For this review, take the finished solid that the model builds, in its own axes (mm). A direction names the side the tool comes from. Give positions to 0.01 mm unless a question says otherwise; leave off trailing zeros. Write each loop counter-clockwise with the first axis right and the second up, starting at its lowest first coordinate (ties: lowest second). Pieces come first, ordered by that corner, then holes. Notation, with made-up numbers: M -25,10.25 L -12,10.25 A23 ccw -12,45.25 Z; hole C 87,-39.5 d10. An arc over 180 degrees is marked long. One line per item, written item: value. Start each with the question number.
Item 1: To check wall thickness, follow probe 1 along X at (y, z) = (95.5, -1); probe 2 along X at (y, z) = (13, -12.5); probe 3 along Y at (x, z) = (33.5, 21.5). State the ranges of each line that lie inside material, in increasing order.
Item 2: Tool access review of faces 3 (the face through (0, 150, 0)), 4 (the face through (6, 0, 30)): name each direction out of +Z, -Z, +X, -X, +Y, -Y from which nothing blocks a thin tool from reaching the whole face with its end or side.
Item 3: Consider section C-C, the plane y = 2. Write out the cut boundary in (x, z).
Item 4: Mouldability with a two-part tool opening along Z and no side actions: class faces 1 (the face through (0, -10, 0)), 2 (the face through (4.336, 65.216, -19.524)) as released by +Z, released by -Z, zero draft, split by the parting line, or undercut.
Item 5: Clearance check with flat-ended pins moving along their axes: pin 1 Ø1 at (y, z) = (36.5, 10.5) entering from -X; pin 2 Ø6 at (y, z) = (40, 7) entering from -X; pin 3 Ø6 at (x, y) = (-21.5, 85.5) entering from +Z. State where each tip first meets the part, or that it passes through.
Item 6: Consider section D-D, the plane y = 40. Write out the cut boundary in (x, z), and give its area (3 significant figures).
```python
from build123d import *

# Parameters (mm, degrees)
F0_R      = 40
F1_DEPTH  = 10
F3_SIZE   = 9.99999
F2_R      = 30
F4_DEPTH  = 10
F5_SIZE   = 9.99999
F6_R      = 20
F7_DEPTH  = 115
F8_SIZE   = 3
F9_R      = 7.5
F10_DEPTH = 25


# Not quite as in the source:
# - a fillet or chamfer is up to 0.001 mm smaller than in the source, because OpenCascade refuses the exact size


with BuildPart() as f1:
    # F0 (on Front) → F1 (new body)
    with BuildSketch(Plane.XZ):
        Circle(F0_R)
    extrude(amount=F1_DEPTH)

    # F3 (size 10 in the source; OpenCascade refuses exactly that, so slightly less here)
    f3_edges = [f1.edges().sort_by_distance(p)[0] for p in [
        (-40, -10, 0),
    ]]
    chamfer(f3_edges, length=F3_SIZE)

    # F2 (on face) → F4 (join)
    with BuildSketch(Plane(origin=(0, 0, 0), x_dir=(-1, 0, 0), z_dir=(0, 1, 0))):
        Circle(F2_R)
    extrude(amount=F4_DEPTH)

    # F5 (size 10 in the source; OpenCascade refuses exactly that, so slightly less here)
    f5_edges = [f1.edges().sort_by_distance(p)[0] for p in [
        (30, 10, 0),
    ]]
    chamfer(f5_edges, length=F5_SIZE)

    # F6 (on face) → F7 (join)
    with BuildSketch(Plane(origin=(0, 10, 0), x_dir=(-1, 0, 0), z_dir=(0, 1, 0))):
        Circle(F6_R)
    extrude(amount=F7_DEPTH)

    # F8
    f8_edges = [f1.edges().sort_by_distance(p)[0] for p in [
        (20, 125, 0),
    ]]
    chamfer(f8_edges, length=F8_SIZE)

    # F9 (on face) → F10 (join)
    with BuildSketch(Plane(origin=(0, 125, 0), x_dir=(-1, 0, 0), z_dir=(0, 1, 0))):
        Circle(F9_R)
    extrude(amount=F10_DEPTH)


solid = f1.part
```
Model answer:
1. probe 1: x = -19.97 to 19.97
1. probe 2: x = -15.61 to 15.61
1. probe 3: y = -0.19 to 0
2. face 3: +Z, -Z, +X, -X, +Y
2. face 4: +Y
3. outline: C 0,0 d56
4. face 1: zero draft
4. face 2: split by the parting line
5. pin 1: stops at x = -17.32
5. pin 2: stops at x = -19.6
5. pin 3: stops at z = 7.6
6. outline: C 0,0 d40
6. area: 1,260 mm2
